Design review of the part shown in the three views and the two pictorial views. Dimensions are in mm from the part's minimum x, y and z. Coordinates: 2 decimals unless noted, no trailing zeros. Write each loop counter-clockwise with the first axis right and the second up, starting at its lowest first coordinate (ties: lowest second). Pieces come first, ordered by that corner, then holes. Notation, with made-up numbers: (-36, 49.5) - (-2, 49.5) arc R20 cw to (-2, 57.5) - close; hole circle Ø8 at (55.25, -9.5). An arc over 180 degrees is marked (long way). Return JSON: item names as keys, results as strings. Group by question number.
(1) To check wall thickness, follow L1, parallel to Z at x = 12, y = 2; L2, parallel to X at y = 7.25, z = 8.25 (1 decimal); L3, parallel to Z at x = 14.5, y = 7.75. State the ranges of each line that lie inside material, in increasing order. Write a range as from..to.
(2) We need section B-B on y = 1.5. State the section outline as (x, z) points.
(3) We need section A-A on y = 4. State the section outline as (x, z) points (1 decimal).
(4) For pin 1 Ø1.5 at (x, z) = (17, 18.5) entering from +Y; pin 2 Ø9.5 at (x, z) = (15.01, 13) entering from +Y, all flat-tipped, find the tip position at first contact; note any pin that passes through.
(5) Draft analysis for pull direction Z (two halves, no side actions). For the marked faces 1, 2 and 3, state which applies: released by +Z, released by -Z, zero draft, split by the parting line, or undercut.
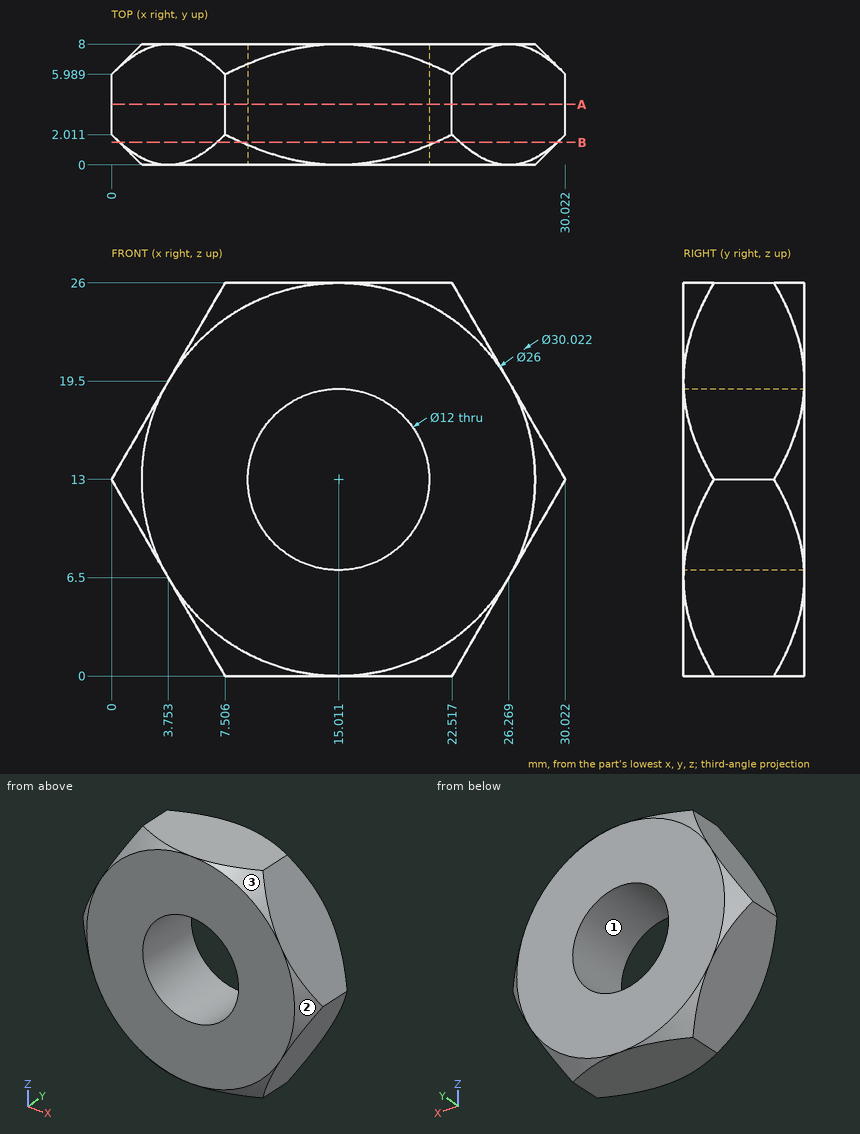
Ans:
{
 "1": {"L1": "0..7.81, 18.19..26", "L2": "2.7..11.3, 18.7..27.3", "L3": "0..7.02, 18.98..26"},
 "2": {"outline": "(0.54, 12.06) - (6.96, 0.94) arc R14.5 ccw to (8.59, 0) - (21.43, 0) arc R14.5 ccw to (23.06, 0.94) - (29.48, 12.06) arc R14.5 ccw to (29.48, 13.94) - (23.06, 25.06) arc R14.5 ccw to (21.43, 26) - (8.59, 26) arc R14.5 ccw to (6.96, 25.06) - (0.54, 13.94) arc R14.5 ccw to start; hole circle Ø12 at (15.01, 13)"},
 "3": {"outline": "(0, 13) - (7.5, 0) - (22.5, 0) - (30, 13) - (22.5, 26) - (7.5, 26) - close; hole circle Ø12 at (15, 13)"},
 "4": {"pin 1": "y = 8", "pin 2": "through"},
 "5": {"face 1": "undercut", "face 2": "split by the parting line", "face 3": "released by +Z"}
}
